from build123d import *

# Parameters (mm, degrees)
SKETCH_2_W          = 40
SKETCH_2_H          = 13
EXTRUDE_1_DEPTH     = 9.5
SKETCH_3_R          = 1
CUT_EXTRUDE_1_DEPTH = 10
SKETCH_4_R          = 1
SKETCH_4_W          = 13
SKETCH_4_H          = 4
CUT_EXTRUDE_2_DEPTH = 10
SKETCH_5_W          = 7
SKETCH_5_H          = 13
CUT_EXTRUDE_3_DEPTH = 5
FILLET_1_R          = 3
EXTRUDE_START       = 1
SKETCH_6_R          = 1
EXTRUDE_2_DEPTH     = 1


with BuildPart() as part:
    # 草图2 → 凸台-拉伸1 (new body)
    with BuildSketch(Plane.XY):
        Rectangle(SKETCH_2_W, SKETCH_2_H)
    extrude(amount=EXTRUDE_1_DEPTH)

    # 草图3 → 切除-拉伸1 (cut)
    with BuildSketch(Plane(origin=(0, 0, 0), x_dir=(-1, 0, 0), z_dir=(0, 0, -1))):
        with Locations((-17.5, 1.5)):
            Circle(SKETCH_3_R)
        with Locations(Location((17.5, 1.5, 0), (0, 0, 180))):
            Circle(SKETCH_3_R)
    extrude(amount=-CUT_EXTRUDE_1_DEPTH, mode=Mode.SUBTRACT)

    # 草图4 → 切除-拉伸2 (cut)
    with BuildSketch(Plane(origin=(0, 0, 0), x_dir=(-1, 0, 0), z_dir=(0, 0, -1))):
        with Locations((-10.7, 4.5)):
            Circle(SKETCH_4_R)
        with Locations(Location((10.7, 4.5, 0), (0, 0, 180))):
            Circle(SKETCH_4_R)
        with Locations((0, 4.5)):
            Rectangle(SKETCH_4_W, SKETCH_4_H)
    extrude(amount=-CUT_EXTRUDE_2_DEPTH, mode=Mode.SUBTRACT)

    # 草图5 → 切除-拉伸3 (cut)
    with BuildSketch(Plane(origin=(0, 0, 0), x_dir=(-1, 0, 0), z_dir=(0, 0, -1))):
        with Locations((-16.5, 0)):
            Rectangle(SKETCH_5_W, SKETCH_5_H)
        with Locations((16.5, 0)):
            Rectangle(SKETCH_5_W, SKETCH_5_H)
    extrude(amount=-CUT_EXTRUDE_3_DEPTH, mode=Mode.SUBTRACT)

    # 圆角1
    fillet_1_edges = [part.edges().sort_by_distance(p)[0] for p in [
        (13, 0, 5),
        (-13, 0, 5),
    ]]
    fillet(fillet_1_edges, radius=FILLET_1_R)

    # 草图6 → 凸台-拉伸2 (add)
    with BuildSketch(Plane(origin=(0, 0, 0), x_dir=(-1, 0, 0), z_dir=(0, 0, -1)).offset(EXTRUDE_START)):
        Polygon((-13, -2.5), (13, -2.5), (13, 6.5), (6.5, 6.5), (6.5, 2.5), (-6.5, 2.5), (-6.5, 6.5), (-13, 6.5), align=None)
        with Locations((-10.7, 4.5)):
            Circle(SKETCH_6_R, mode=Mode.SUBTRACT)
        with Locations((10.7, 4.5)):
            Circle(SKETCH_6_R, mode=Mode.SUBTRACT)
    extrude(amount=-EXTRUDE_2_DEPTH)


solid = part.part
Could you check a few things on this model? Use its own coordinates, in mm. A direction names the side the tool comes from. Give positions to 0.01 mm unless a question says otherwise; leave off trailing zeros. Order: outer loops, then holes, each group sorted by start corner. A loop starts at its lowest first (then second) coordinate and runs counter-clockwise, first axis right, second up. Notation, with made-up numbers: (45, -19.5) - (63, -19.5) arc R27 ccw to (63, 14.5) - close; hole circle Ø8 at (58, -25). An arc over 180 degrees is marked (long way). One line per item, written item: value. Start each with the question number.
1. Imagine slicing it at D-D on z = 6.5. List the corners of the cut face in (x, y) for me, plus the area to 3 significant figures.
2. Imagine slicing it at A-A on x = -17.5. List the corners of the cut face in (y, z) for me, plus the area to 3 significant figures.
3. For faces 4 (the face through (-13, 0, 0)), 5 (the face through (0, 2.5, 4)), 6 (the face through (16.576, 1.117, 7.219)), 7 (the face through (18, 0, 5)), 8 (the face through (0, -4, 0)), which set-ups out of +Z, -Z, +X, -X, +Y, -Y let a thin tool reach every point of the face, with its end or its side?
4. Imagine slicing it at B-B on y = 4.5. List the corners of the cut face in (x, z) for me.
5. Thinking about a two-plate mould opening in X: for faces 1 (the face through (-18, 0, 5)), 2 (the face through (-20, 0, 7)), 3 (the face through (-6.5, 5, 4)), which applies, +X half, -X half, draft (parallel to the pull), parting line (faces both ways), or undercut?
6. Imagine slicing it at C-C on y = 1.5. List the corners of the cut face in (x, z) for me.
7. If I drill on probe 1 along Y at (x, z) = (-10.7, 6.75); probe 2 along Y at (x, z) = (-17.5, 6.65); probe 3 along X at (y, z) = (6, 1.75), over which ranges is the centre line in solid material (lowest first)?
8. For P1, Ø5, axis at y = -4, z = 3.5, coming from the -X side; P2, Ø3, axis at x = 17, y = -1, coming from the -Z side; P3, Ø2, axis at y = -1, z = 0, coming from the +X side; P4, Ø0.5, axis at x = -3.5, z = -0.5, coming from the -Y side, each with a flat end and sliding along its axis, tell me the tip position at first contact or that it passes through.
Values:
1. outline: (-20, -6.5) - (20, -6.5) - (20, 6.5) - (6.5, 6.5) - (6.5, 2.5) - (-6.5, 2.5) - (-6.5, 6.5) - (-20, 6.5) - close; hole circle Ø2 at (-17.5, 1.5); hole circle Ø2 at (-10.7, 4.5); hole circle Ø2 at (10.7, 4.5); hole circle Ø2 at (17.5, 1.5)
1. area: 455 mm²
2. outline: (-6.5, 5) - (0.5, 5) - (0.5, 9.5) - (-6.5, 9.5) - close; (2.5, 5) - (6.5, 5) - (6.5, 9.5) - (2.5, 9.5) - close
2. area: 49.5 mm²
3. face 4: -Z, -X, +Y, -Y
3. face 5: +Z, -Z, +Y
3. face 6: +Z, -Z
3. face 7: -Z, +X, +Y, -Y
3. face 8: -Z, +X, -X, -Y
4. outline: (-20, 5) - (-16, 5) arc R3 cw to (-13, 2) - (-13, -1) - (-11.7, -1) - (-11.7, 9.5) - (-20, 9.5) - close; (-9.7, -1) - (-6.5, -1) - (-6.5, 9.5) - (-9.7, 9.5) - close; (6.5, -1) - (9.7, -1) - (9.7, 9.5) - (6.5, 9.5) - close; (11.7, -1) - (13, -1) - (13, 2) arc R3 cw to (16, 5) - (20, 5) - (20, 9.5) - (11.7, 9.5) - close
5. face 1: draft
5. face 2: -X half
5. face 3: undercut
6. outline: (-20, 5) - (-18.5, 5) - (-18.5, 9.5) - (-20, 9.5) - close; (-16.5, 5) - (-16, 5) arc R3 cw to (-13, 2) - (-13, -1) - (13, -1) - (13, 2) arc R3 cw to (16, 5) - (16.5, 5) - (16.5, 9.5) - (-16.5, 9.5) - close; (18.5, 5) - (20, 5) - (20, 9.5) - (18.5, 9.5) - close
7. probe 1: -6.5 to 3.5, 5.5 to 6.5
7. probe 2: -6.5 to 0.5, 2.5 to 6.5
7. probe 3: -13 to -6.5, 6.5 to 13
8. P1: x = -20
8. P2: z = 4.96
8. P3: x = 13
8. P4: y = -2.5
